Can you work these out from the model? Positions are in its coordinate system, mm. A direction names the side the tool comes from. Coordinates: 2 decimals unless noted, no trailing zeros. Loops run counter-clockwise (first coordinate to the right, second up) from the corner with the lowest first, then second, coordinate; pieces in that order, holes last.
```python
from build123d import *

# Parameters (mm, degrees)
F0_R     = 2.25
F1_DEPTH = 4.330125
F2_R     = 5.8
F4_DEPTH = 28
F5_R     = 2.25
F6_DEPTH = 25


with BuildPart() as f1:
    # F0 (on Top) → F1 (new body, symmetric)
    with BuildSketch(Plane.XY):
        Polygon((-7.5, 47.100404), (0, 27.485359), (0, 58.922307), (-5.601237, 73.922307), (-12.020218, 73.922307), (-12.020218, 58.922307), (-9.755767, 53), (-7.5, 53), align=None)
        with Locations((-9.75, 66.422307)):
            Circle(F0_R, mode=Mode.SUBTRACT)
    extrude(amount=F1_DEPTH, both=True)

    # F2
    f2_edges = [f1.edges().sort_by_distance(p)[0] for p in [
        (-5.601237, 73.922307, 0),
    ]]
    fillet(f2_edges, radius=F2_R)

    # F3 (on face) → F4 (join)
    with BuildSketch(Plane(origin=(-12.020218, 0, 0), x_dir=(0, -1, 0), z_dir=(-1, 0, 0))):
        Polygon((-70.466645, -2.501664), (-71.522307, -4.330125), (-66.722307, -4.330125), (-67.777969, -2.501664), align=None)
    extrude(amount=F4_DEPTH)

    # F5 (on face) → F6 (cut)
    with BuildSketch(Plane.XY.offset(4.330125)):
        with Locations((-30.15, 66.422307)):
            Circle(F5_R)
    extrude(amount=-F6_DEPTH, mode=Mode.SUBTRACT)


solid = f1.part
```
(1) I want a section at A-A on z = 1. Write out the boundary of the cut face in (x, y), then the cut area to 3 significant figures.
Check values:
outline: (-12.02, 58.92) - (-9.76, 53) - (-7.5, 53) - (-7.5, 47.1) - (0, 27.49) - (0, 58.92) - (-4.19, 70.15) arc R5.8 ccw to (-9.63, 73.92) - (-12.02, 73.92) - close; hole circle Ø4.5 at (-9.75, 66.42)
area: 302 mm2
(2) Which directions (+Z, -Z, +X, -X, +Y, -Y) give clear straight access to the entire face, cutting with the end or side of a thin tool? Please do faces 1 (the flat face through (-25.824, 70.987, -3.403)), 2 (the flat face through (-20.07, 67.24, -3.43)), 3 (the flat face through (-26, 69, -2.502)), 4 (the flat face through (-7.5, 50, 0)), 5 (the cylindrical face through (-6.36, 72.915, 0.061)).
Check values:
face 1: +Z, -X, +Y
face 2: +Z, -X, -Y
face 3: +Z, -X, +Y, -Y
face 4: +Z, -Z, -X, -Y
face 5: +Z, -Z, +X, +Y
(3) If I drill on probe 1 along X at (y, z) = (50, 1.5); probe 2 along Z at (x, y) = (-18, 69.5); probe 3 along X at (y, z) = (34, -3), over which ranges is the centre line in solid material (lowest first)?
Check values:
probe 1: x = -7.5 to 0
probe 2: z = -4.33 to -2.5
probe 3: x = -2.49 to 0
(4) If we mould it in two halves opening along X, with no side actions, what happens to faces 6 (the cylindrical face through (-10.043, 68.653, -0.061)), 7 (the flat face through (-9, 53, 0)), 8 (the flat face through (-3.802, 37.43, 0.061)), 9 (the flat face through (0, 43, 0))? For each: released by +X, released by -X, zero draft, split by the parting line, or undercut.
Check values:
face 6: undercut
face 7: zero draft
face 8: released by -X
face 9: released by +X
(5) I'm going to push flat-ended pins straight in: pin 1 (1.1 mm diameter, centred on x = -8.5, z = -0.5, fed in from -Y); pin 2 (0.8 mm diameter, centred on x = -29.5, y = 69, fed in from +Z); pin 3 (3 mm diameter, centred on y = 50.5, z = 1, fed in from -X). Where does each tip first touch, or does it pass through?
Check values:
pin 1: stops at y = 53
pin 2: stops at z = -2.5
pin 3: stops at x = -7.5
(6) I want a section at C-C on y = 49. Write out the boundary of the cut face in (x, z), then the cut area to 3 significant figures.
Check values:
outline: (-7.5, -4.33) - (0, -4.33) - (0, 4.33) - (-7.5, 4.33) - close
area: 65.0 mm2
(7) I want a section at B-B on x = -33. Write out the boundary of the cut face in (y, z).
Check values:
outline: (66.72, -4.33) - (71.52, -4.33) - (70.47, -2.5) - (67.78, -2.5) - close
